The model under review builds one solid part; all positions refer to its coordinate system, in mm. Face numbers are marked on the shaded views. A direction names the side the tool comes from. Round coordinates to 2 decimals unless told otherwise and drop trailing zeros. Write each loop counter-clockwise with the first axis right and the second up, starting at its lowest first coordinate (ties: lowest second). Pieces come first, ordered by that corner, then holes.
Item 1: Machinability: for the marked faces 1, 2, 3 and 4, which of the approach directions +Z, -Z, +X, -X, +Y, -Y give a long, thin tool a straight path to every point of the face, cutting with its end or side? Answer none if there is none.
Item 2: Add section B-B (z = -0.5). Give the boundary of the cut face in (x, y), plus the area to 3 significant figures.
Item 3: Add section C-C (z = 1.5). Give the boundary of the cut face in (x, y), plus the area to 3 significant figures.
Item 4: Clearance check with flat-ended pins moving along their axes: pin 1 Ø1.1 at (x, y) = (2, -1.5) entering from +Z; pin 2 Ø2 at (x, z) = (13, 2.5) entering from -Y; pin 3 Ø1.5 at (x, z) = (0.5, -1) entering from +Y. State where each tip first meets the part, or that it passes through.
Item 5: To check wall thickness, follow L1, parallel to Y at x = 9.5, z = 0.25; L2, parallel to Y at x = 14, z = 0.45; L3, parallel to Y at x = 0, z = 2.75. State the ranges of each line that lie inside material, in increasing order.
Item 6: Draft analysis for pull direction X (two halves, no side actions). For the marked faces 5, 6 and 7, state which applies: +X half, -X half, draft (parallel to the pull), parting line (faces both ways), or undercut.
Item 7: Add section D-D (x = 3.5). State how many separate pieces and enclosed holes the cut face has, plus the area to 3 significant figures.
Item 8: Add section A-A (z = 3.75). Give the boundary of the cut face in (x, y).
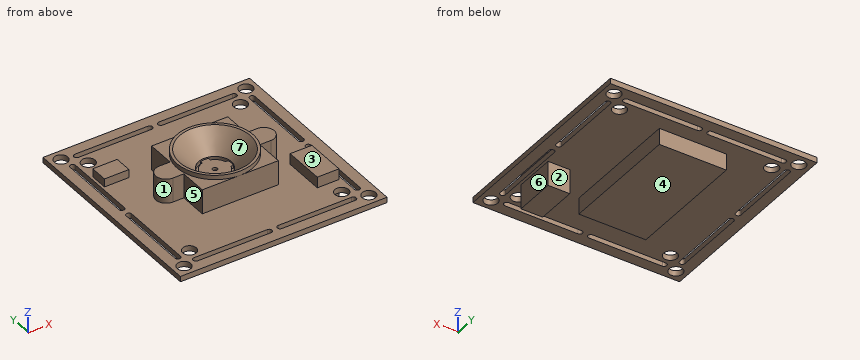
```python
from build123d import *

# Parameters (mm, degrees)
SKETCH_1_W          = 38
SKETCH_1_H          = 38
SKETCH_1_R          = 1.25
EXTRUDE_1_DEPTH     = 1
EXTRUDE_2_DEPTH     = 4.5
SKETCH_3_R          = 7
EXTRUDE_3_DEPTH     = 0.8
CUT_EXTRUDE_START   = -0.5
SKETCH_5_R          = 0.438948094
CUT_EXTRUDE_1_DEPTH = 0.5
SKETCH_6_W          = 12.323185316
SKETCH_6_H          = 22.259619553
EXTRUDE_4_DEPTH     = 3
SKETCH_7_W          = 4
SKETCH_7_H          = 7.5
EXTRUDE_5_DEPTH     = 4.5
SKETCH_9_W          = 4.5
SKETCH_9_H          = 3.25
EXTRUDE_6_DEPTH     = 1.5
SKETCH_10_W         = 4
SKETCH_10_H         = 7.5
EXTRUDE_7_DEPTH     = 2


with BuildPart() as part:
    # ｽｹｯﾁ1 → ﾎﾞｽ - 押し出し1 (new body)
    with BuildSketch(Plane.XY):
        Rectangle(SKETCH_1_W, SKETCH_1_H)
        with Locations((17, 17)):
            Circle(SKETCH_1_R, mode=Mode.SUBTRACT)
        with Locations((14, 14)):
            Circle(SKETCH_1_R, mode=Mode.SUBTRACT)
        with Locations((17, -17)):
            Circle(SKETCH_1_R, mode=Mode.SUBTRACT)
        with Locations((14, -14)):
            Circle(SKETCH_1_R, mode=Mode.SUBTRACT)
        with Locations((-17, -17)):
            Circle(SKETCH_1_R, mode=Mode.SUBTRACT)
        with Locations((-14, -14)):
            Circle(SKETCH_1_R, mode=Mode.SUBTRACT)
        with Locations((-17, 17)):
            Circle(SKETCH_1_R, mode=Mode.SUBTRACT)
        with Locations((-14, 14)):
            Circle(SKETCH_1_R, mode=Mode.SUBTRACT)
        with BuildLine():
            Line((1, 17), (14.5, 17))
            ThreePointArc((14.5, 17), (15, 16.5), (14.5, 16))
            Line((14.5, 16), (1, 16))
            ThreePointArc((1, 16), (0.5, 16.5), (1, 17))
        make_face(mode=Mode.SUBTRACT)
        with BuildLine():
            Line((-1, 17), (-14.5, 17))
            ThreePointArc((-14.5, 17), (-15, 16.5), (-14.5, 16))
            Line((-14.5, 16), (-1, 16))
            ThreePointArc((-1, 16), (-0.5, 16.5), (-1, 17))
        make_face(mode=Mode.SUBTRACT)
        with BuildLine():
            Line((17, -1), (17, -14.5))
            ThreePointArc((17, -14.5), (16.5, -15), (16, -14.5))
            Line((16, -14.5), (16, -1))
            ThreePointArc((16, -1), (16.5, -0.5), (17, -1))
        make_face(mode=Mode.SUBTRACT)
        with BuildLine():
            Line((17, 1), (17, 14.5))
            ThreePointArc((17, 14.5), (16.5, 15), (16, 14.5))
            Line((16, 14.5), (16, 1))
            ThreePointArc((16, 1), (16.5, 0.5), (17, 1))
        make_face(mode=Mode.SUBTRACT)
        with BuildLine():
            Line((-1, -17), (-14.5, -17))
            ThreePointArc((-14.5, -17), (-15, -16.5), (-14.5, -16))
            Line((-14.5, -16), (-1, -16))
            ThreePointArc((-1, -16), (-0.5, -16.5), (-1, -17))
        make_face(mode=Mode.SUBTRACT)
        with BuildLine():
            Line((1, -17), (14.5, -17))
            ThreePointArc((14.5, -17), (15, -16.5), (14.5, -16))
            Line((14.5, -16), (1, -16))
            ThreePointArc((1, -16), (0.5, -16.5), (1, -17))
        make_face(mode=Mode.SUBTRACT)
        with BuildLine():
            Line((-17, 1), (-17, 14.5))
            ThreePointArc((-17, 14.5), (-16.5, 15), (-16, 14.5))
            Line((-16, 14.5), (-16, 1))
            ThreePointArc((-16, 1), (-16.5, 0.5), (-17, 1))
        make_face(mode=Mode.SUBTRACT)
        with BuildLine():
            Line((-17, -1), (-17, -14.5))
            ThreePointArc((-17, -14.5), (-16.5, -15), (-16, -14.5))
            Line((-16, -14.5), (-16, -1))
            ThreePointArc((-16, -1), (-16.5, -0.5), (-17, -1))
        make_face(mode=Mode.SUBTRACT)
    extrude(amount=EXTRUDE_1_DEPTH)

    # ｽｹｯﾁ2 → ﾎﾞｽ - 押し出し2 (add)
    with BuildSketch(Plane.XY.offset(1)):
        with BuildLine():
            Line((-7, -7), (7, -7))
            Line((7, -7), (7, -1.896601527))
            Line((7, -1.896601527), (9, -1.896601527))
            ThreePointArc((9, -1.896601527), (10.896601527, 0), (9, 1.896601527))
            Line((9, 1.896601527), (7, 1.896601527))
            Line((7, 1.896601527), (7, 7))
            Line((7, 7), (-7, 7))
            Line((-7, 7), (-7, 1.896601527))
            Line((-7, 1.896601527), (-9, 1.896601527))
            ThreePointArc((-9, 1.896601527), (-10.896601527, 0), (-9, -1.896601527))
            Line((-9, -1.896601527), (-7, -1.896601527))
            Line((-7, -1.896601527), (-7, -7))
        make_face()
    extrude(amount=EXTRUDE_2_DEPTH)

    # ｽｹｯﾁ3 → ﾎﾞｽ - 押し出し3 (add)
    with BuildSketch(Plane.XY.offset(5.5)):
        with Locations(Location((0, 0, 0), (0, 0, 270))):
            Circle(SKETCH_3_R)
    extrude(amount=EXTRUDE_3_DEPTH)

    # ｽｹｯﾁ4 → ｶｯﾄ - 回転1 (revolve, cut)
    with BuildSketch(Plane(origin=(0, 0, 0), x_dir=(1, 0, 0), z_dir=(0, 1, 0))):
        Polygon((-6.5, -6.3), (-3, -2.8), (-3, -2.55), (0, -2.55), (0, -6.3), align=None)
    revolve(axis=Axis((0, 0, 0), (0, 0, 1)), mode=Mode.SUBTRACT)

    # ｽｹｯﾁ5 → ｶｯﾄ - 押し出し1 (cut)
    with BuildSketch(Plane.XY.offset(2.55).offset(CUT_EXTRUDE_START)):
        Circle(SKETCH_5_R)
        with BuildLine():
            Line((0.75, 2.90473751), (0.75, 2.431581232))
            ThreePointArc((0.75, 2.431581232), (1.79931755, 1.79931755), (2.431581232, 0.75))
            Line((2.431581232, 0.75), (2.90473751, 0.75))
            ThreePointArc((2.90473751, 0.75), (2.121320344, 2.121320344), (0.75, 2.90473751))
        make_face()
        with BuildLine():
            Line((2.90473751, -0.75), (2.431581232, -0.75))
            ThreePointArc((2.431581232, -0.75), (1.79931755, -1.79931755), (0.75, -2.431581232))
            Line((0.75, -2.431581232), (0.75, -2.90473751))
            ThreePointArc((0.75, -2.90473751), (2.121320344, -2.121320344), (2.90473751, -0.75))
        make_face()
        with BuildLine():
            Line((-0.75, -2.90473751), (-0.75, -2.431581232))
            ThreePointArc((-0.75, -2.431581232), (-1.79931755, -1.79931755), (-2.431581232, -0.75))
            Line((-2.431581232, -0.75), (-2.90473751, -0.75))
            ThreePointArc((-2.90473751, -0.75), (-2.121320344, -2.121320344), (-0.75, -2.90473751))
        make_face()
        with BuildLine():
            Line((-2.90473751, 0.75), (-2.431581232, 0.75))
            ThreePointArc((-2.431581232, 0.75), (-1.79931755, 1.79931755), (-0.75, 2.431581232))
            Line((-0.75, 2.431581232), (-0.75, 2.90473751))
            ThreePointArc((-0.75, 2.90473751), (-2.121320344, 2.121320344), (-2.90473751, 0.75))
        make_face()
    extrude(amount=CUT_EXTRUDE_1_DEPTH, mode=Mode.SUBTRACT)

    # ｽｹｯﾁ6 → ﾎﾞｽ - 押し出し4 (add)
    with BuildSketch(Plane(origin=(0, 0, 0), x_dir=(-1, 0, 0), z_dir=(0, 0, -1))):
        with Locations((0, 2.099913023)):
            Rectangle(SKETCH_6_W, SKETCH_6_H)
    extrude(amount=EXTRUDE_4_DEPTH)

    # ｽｹｯﾁ7 → ﾎﾞｽ - 押し出し5 (add)
    with BuildSketch(Plane(origin=(0, 0, 0), x_dir=(-1, 0, 0), z_dir=(0, 0, -1))):
        with Locations((-13.5, -7.25)):
            Rectangle(SKETCH_7_W, SKETCH_7_H)
    extrude(amount=EXTRUDE_5_DEPTH)

    # ｽｹｯﾁ9 → ﾎﾞｽ - 押し出し6 (add)
    with BuildSketch(Plane.XY.offset(1)):
        with Locations((-13.25, 8.875)):
            Rectangle(SKETCH_9_W, SKETCH_9_H)
    extrude(amount=EXTRUDE_6_DEPTH)

    # ｽｹｯﾁ10 → ﾎﾞｽ - 押し出し7 (add)
    with BuildSketch(Plane.XY.offset(1)):
        with Locations((13.5, -7.25)):
            Rectangle(SKETCH_10_W, SKETCH_10_H)
    extrude(amount=EXTRUDE_7_DEPTH)


solid = part.part
```
Numbers:
1. face 1: +Z, -X
1. face 2: -Z, +X, +Y
1. face 3: +Z, +X, +Y, -Y
1. face 4: -Z, -X, +Y, -Y
2. outline: (-6.16, -9.03) - (6.16, -9.03) - (6.16, 13.23) - (-6.16, 13.23) - close; (11.5, -11) - (15.5, -11) - (15.5, -3.5) - (11.5, -3.5) - close
2. area: 304 mm2
3. outline: (-15.5, 7.25) - (-11, 7.25) - (-11, 10.5) - (-15.5, 10.5) - close; (-9, -1.9) - (-7, -1.9) - (-7, -7) - (7, -7) - (7, -1.9) - (9, -1.9) arc R1.9 ccw to (9, 1.9) - (7, 1.9) - (7, 7) - (-7, 7) - (-7, 1.9) - (-9, 1.9) arc R1.9 ccw to start; (11.5, -11) - (15.5, -11) - (15.5, -3.5) - (11.5, -3.5) - close
3. area: 267 mm2
4. pin 1: stops at z = 2.85
4. pin 2: stops at y = -11
4. pin 3: stops at y = 13.23
5. L1: y = -19 to -17, -16 to 16, 17 to 19
5. L2: y = -19 to -17, -16 to -15.25, -12.75 to 12.75, 15.25 to 16, 17 to 19
5. L3: y = -7 to -3, 3 to 7
6. face 5: -X half
6. face 6: +X half
6. face 7: undercut
7. separate pieces: 3
7. enclosed holes: 0
7. area: 155 mm2
8. outline: (-9, -1.9) - (-7, -1.9) - (-7, -7) - (7, -7) - (7, -1.9) - (9, -1.9) arc R1.9 ccw to (9, 1.9) - (7, 1.9) - (7, 7) - (-7, 7) - (-7, 1.9) - (-9, 1.9) arc R1.9 ccw to start; hole circle Ø7.9 at (0, 0)
